```python
from build123d import *

# Parameters (mm, degrees)
SKETCH_3_R          = 17
EXTRUDE_2_DEPTH     = 8
SKETCH_6_W          = 34
SKETCH_6_H          = 15
EXTRUDE_3_DEPTH     = 8
SKETCH_4_R          = 13
CUT_EXTRUDE_1_DEPTH = 8
SKETCH_5_W          = 39.282271498
SKETCH_5_H          = 26.093650735
CUT_EXTRUDE_2_DEPTH = 8


with BuildPart() as part:
    # 스케치3 → 보스-돌출2 (new body)
    with BuildSketch(Plane(origin=(0, 0, 0), x_dir=(1, 0, 0), z_dir=(0, 1, 0))):
        Circle(SKETCH_3_R)
    extrude(amount=EXTRUDE_2_DEPTH)

    # 스케치6 → 보스-돌출3 (add)
    with BuildSketch(Plane(origin=(0, 8, 0), x_dir=(1, 0, 0), z_dir=(0, 1, 0))):
        with Locations((0, -7.5)):
            Rectangle(SKETCH_6_W, SKETCH_6_H)
    extrude(amount=-EXTRUDE_3_DEPTH)

    # 스케치4 → 컷-돌출1 (cut)
    with BuildSketch(Plane(origin=(0, 8, 0), x_dir=(1, 0, 0), z_dir=(0, 1, 0))):
        Circle(SKETCH_4_R)
    extrude(amount=-CUT_EXTRUDE_1_DEPTH, mode=Mode.SUBTRACT)

    # 스케치5 → 컷-돌출2 (cut)
    with BuildSketch(Plane(origin=(0, 8, 0), x_dir=(1, 0, 0), z_dir=(0, 1, 0))):
        with Locations((-0.462251139, 5.046825368)):
            Rectangle(SKETCH_5_W, SKETCH_5_H)
    extrude(amount=-CUT_EXTRUDE_2_DEPTH, mode=Mode.SUBTRACT)


solid = part.part
```
For this review, take the finished solid that the model builds, in its own axes (mm). A direction names the side the tool comes from. Coordinates: 2 decimals unless noted, no trailing zeros. Write each loop counter-clockwise with the first axis right and the second up, starting at its lowest first coordinate (ties: lowest second). Pieces come first, ordered by that corner, then holes. Notation, with made-up numbers: (82.25, 48.5) - (128.25, 48.5) arc R20 ccw to (128.25, 76.5) - close; hole circle Ø3 at (42, 7.25). An arc over 180 degrees is marked (long way). Answer in a Markdown table with one row per item. Add a question column.
Q1. We need section B-B, the plane y = 4.5. State the section outline as (x, z) points, and give its area (3 significant figures).
Q2. We need section D-D, the plane x = -13. State the section outline as (y, z) points.
Q3. Tool access review of faces 4 (the flat face through (14, 4, 8)), 5 (the flat face through (-13, 4, 15)): name each direction out of +Z, -Z, +X, -X, +Y, -Y from which nothing blocks a thin tool from reaching the whole face with its end or side.
Q4. For P1, Ø1, axis at x = -9, y = 4.5, coming from the +Z side; P2, Ø3, axis at x = -12.5, z = 13, coming from the -Y side, all flat-tipped, find the tip position at first contact; note any pin that passes through.
Q5. We need section A-A, the plane z = 12. State the section outline as (x, y) points.
Q6. For probe 1 along X at (y, z) = (5.5, 11); probe 2 along X at (y, z) = (6.75, 10.5); probe 3 along Z at (x, y) = (-15, 7.5), list the stretches that pass through material, from the lowest coordinate up.
Q7. Draft analysis for pull direction X (two halves, no side actions). For faces 1 (the cylindrical face through (0, 4, 13)), 2 (the flat face through (12, 4, 15)), 3 (the cylindrical face through (0, 4, 17)), state which applies: +X half, -X half, draft (parallel to the pull), parting line (faces both ways), or undercut.
Q8. We need section C-C, the plane z = 10.25. State the section outline as (x, y) points.
Answer list:
| question | item | result |
|---|---|---|
| 1 | outline | (-17, 8) - (-10.25, 8) arc R13 cw to (10.25, 8) - (17, 8) - (17, 15) - (8, 15) arc R17 ccw to (-8, 15) - (-17, 15) - close |
| 1 | area | 188 mm2 |
| 2 | outline | (0, 8) - (8, 8) - (8, 15) - (0, 15) - close |
| 3 | face 4 | -Z, +X, -X, +Y, -Y |
| 3 | face 5 | +Z, -X, +Y, -Y |
| 4 | P1 | stops at z = 15 |
| 4 | P2 | stops at y = 0 |
| 5 | outline | (-17, 0) - (-5, 0) - (-5, 8) - (-17, 8) - close; (5, 0) - (17, 0) - (17, 8) - (5, 8) - close |
| 6 | probe 1 | x = -17 to -6.93, 6.93 to 17 |
| 6 | probe 2 | x = -17 to -7.66, 7.66 to 17 |
| 6 | probe 3 | z = 8 to 15 |
| 7 | face 1 | undercut |
| 7 | face 2 | draft |
| 7 | face 3 | parting line |
| 8 | outline | (-17, 0) - (-8, 0) - (-8, 8) - (-17, 8) - close; (8, 0) - (17, 0) - (17, 8) - (8, 8) - close |
